Source: CAD feature listing. Evaluate the final solid. Frame: model axes, mm. Give positions to 0.01 mm unless a question says otherwise; leave off trailing zeros. Order: outer loops, then holes, each group sorted by start corner. A loop starts at its lowest first (then second) coordinate and runs counter-clockwise, first axis right, second up. Notation, with made-up numbers: M 81,80.5 L 96,80.5 A22 cw 96,116.5 Z; hole C 54.25,79.25 d1. An arc over 180 degrees is marked long. Return JSON: item names as keys, results as strings.
from build123d import *

# Parameters (mm, degrees)
SKETCH1_W           = 203.2
SKETCH1_H           = 127
BOSS_EXTRUDE1_DEPTH = 10
SKETCH2_R           = 2.49
CUT_EXTRUDE1_DEPTH  = 10


with BuildPart() as part:
    # Sketch1 → Boss-Extrude1 (new body)
    with BuildSketch(Plane.XY):
        with Locations((-101.6, -63.5)):
            Rectangle(SKETCH1_W, SKETCH1_H)
    extrude(amount=BOSS_EXTRUDE1_DEPTH)

    # Sketch2 → Cut-Extrude1 (cut)
    with BuildSketch(Plane.XY.offset(10)):
        with Locations((-177.8, -25.4)):
            Circle(SKETCH2_R)
        with Locations((-152.4, -25.4)):
            Circle(SKETCH2_R)
        with Locations((-127, -25.4)):
            Circle(SKETCH2_R)
        with Locations((-101.6, -25.4)):
            Circle(SKETCH2_R)
        with Locations((-76.2, -25.4)):
            Circle(SKETCH2_R)
        with Locations((-50.8, -25.4)):
            Circle(SKETCH2_R)
        with Locations((-25.4, -25.4)):
            Circle(SKETCH2_R)
        with Locations((-152.4, -50.8)):
            Circle(SKETCH2_R)
        with Locations((-127, -50.8)):
            Circle(SKETCH2_R)
        with Locations((-101.6, -50.8)):
            Circle(SKETCH2_R)
        with Locations((-76.2, -50.8)):
            Circle(SKETCH2_R)
        with Locations((-50.8, -50.8)):
            Circle(SKETCH2_R)
        with Locations((-25.4, -50.8)):
            Circle(SKETCH2_R)
        with Locations((-152.4, -76.2)):
            Circle(SKETCH2_R)
        with Locations((-127, -76.2)):
            Circle(SKETCH2_R)
        with Locations((-101.6, -76.2)):
            Circle(SKETCH2_R)
        with Locations((-76.2, -76.2)):
            Circle(SKETCH2_R)
        with Locations((-50.8, -76.2)):
            Circle(SKETCH2_R)
        with Locations((-25.4, -76.2)):
            Circle(SKETCH2_R)
        with Locations((-152.4, -101.6)):
            Circle(SKETCH2_R)
        with Locations((-127, -101.6)):
            Circle(SKETCH2_R)
        with Locations((-101.6, -101.6)):
            Circle(SKETCH2_R)
        with Locations((-76.2, -101.6)):
            Circle(SKETCH2_R)
        with Locations((-50.8, -101.6)):
            Circle(SKETCH2_R)
        with Locations((-25.4, -101.6)):
            Circle(SKETCH2_R)
        with Locations((-177.8, -50.8)):
            Circle(SKETCH2_R)
        with Locations((-177.8, -76.2)):
            Circle(SKETCH2_R)
        with Locations((-177.8, -101.6)):
            Circle(SKETCH2_R)
    extrude(amount=-CUT_EXTRUDE1_DEPTH, mode=Mode.SUBTRACT)


solid = part.part
1. Ray query, probe 1 along Y at (x, z) = (-25.4, 2.75); probe 2 along Y at (x, z) = (-153.5, 7). Return the intervals inside material, ascending.
Evaluation:
{"probe 1": "y = -127 to -104.09, -99.11 to -78.69, -73.71 to -53.29, -48.31 to -27.89, -22.91 to 0", "probe 2": "y = -127 to -103.83, -99.37 to -78.43, -73.97 to -53.03, -48.57 to -27.63, -23.17 to 0"}
2. First-contact query: pin 1 (1 mm diameter, centred on y = -113, z = 4, fed in from +X). Flat tip, straight axial feed; report the tip coordinate or a pass-through.
Evaluation:
{"pin 1": "stops at x = 0"}
3. Section query A-A (x = -177.8). Return loops of the section in (y, z), then the cut area to 3 significant figures.
Evaluation:
{"outline": "M -127,0 L -104.09,0 L -104.09,10 L -127,10 Z; M -99.11,0 L -78.69,0 L -78.69,10 L -99.11,10 Z; M -73.71,0 L -53.29,0 L -53.29,10 L -73.71,10 Z; M -48.31,0 L -27.89,0 L -27.89,10 L -48.31,10 Z; M -22.91,0 L 0,0 L 0,10 L -22.91,10 Z", "area": "1,070 mm^2"}
4. Draft query along X for faces 1 (the face through (-25.94, -53.23, 5.07)), 2 (the face through (0, -64, 5)), 3 (the face through (-154.376, -77.715, 5.07)), 4 (the face through (-103, -127, 5)). Return one class per face: pulls with the +X half, pulls with the -X half, needs draft (parallel to the pull), parting line crosses it, or undercut.
Evaluation:
{"face 1": "undercut", "face 2": "pulls with the +X half", "face 3": "undercut", "face 4": "needs draft"}
5. Section query B-B (y = -50.8). State how many separate pieces and enclosed holes the cut face has, then the cut area to 3 significant figures.
Evaluation:
{"separate pieces": "8", "enclosed holes": "0", "area": "1,680 mm^2"}
